Design review of the part shown in the three views and the two pictorial views. Dimensions are in mm from the part's minimum x, y and z. A direction names the side the tool comes from. Round coordinates to 2 decimals unless told otherwise and drop trailing zeros. Write each loop counter-clockwise with the first axis right and the second up, starting at its lowest first coordinate (ties: lowest second). Pieces come first, ordered by that corner, then holes. Notation, with made-up numbers: (30, 53.25) - (56, 53.25) arc R33 cw to (56, 89.25) - close; hole circle Ø5 at (25.25, 20.5). An arc over 180 degrees is marked (long way). Use one line per item in the form item = value.
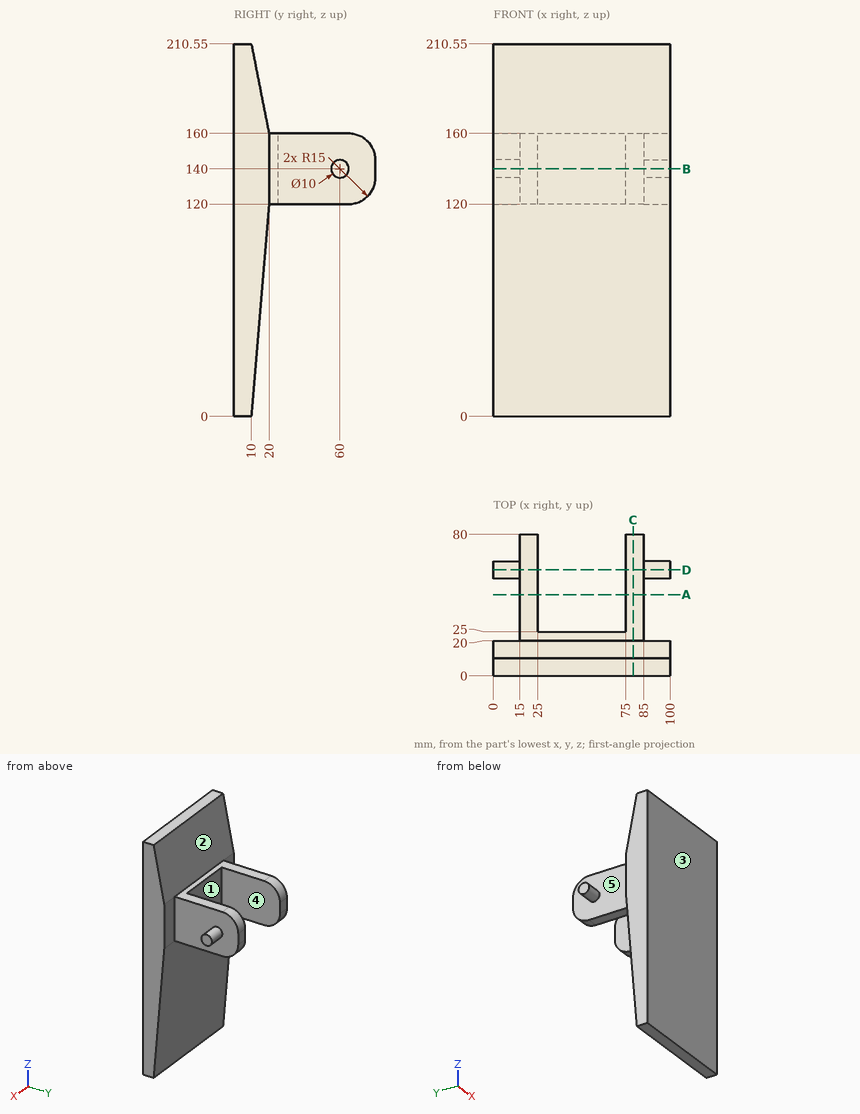
Q1. We need section C-C on x = 79. Write out the cut boundary in (y, z).
Calculated:
outline = (0, 0) - (10, 0) - (20, 120) - (65, 120) arc R15 ccw to (80, 135) - (80, 145) arc R15 ccw to (65, 160) - (20, 160) - (10, 210.55) - (0, 210.55) - close
Q2. To check wall thickness, follow line 1 along X through (y, z) = (32, 128.5); line 2 along Y through (x, z) = (50, 155.5); line 3 along Z through (x, y) = (20.5, 37). State the ranges of each line that lie inside material, in increasing order. Write a range as from..to.
Calculated:
line_1 = 15..25, 75..85
line_2 = 0..25
line_3 = 120..160
Q3. We need section A-A on y = 46. Write out the cut boundary in (x, z).
Calculated:
outline = (15, 120) - (25, 120) - (25, 160) - (15, 160) - close; (75, 120) - (85, 120) - (85, 160) - (75, 160) - close
Q4. We need section D-D on y = 60. Write out the cut boundary in (x, z).
Calculated:
outline = (0, 135) - (15, 135) - (15, 120) - (25, 120) - (25, 160) - (15, 160) - (15, 145) - (0, 145) - close; (75, 120) - (85, 120) - (85, 135) - (100, 135) - (100, 145) - (85, 145) - (85, 160) - (75, 160) - close
Q5. Machinability: for the marked faces 1 and 2, which of the approach directions +Z, -Z, +X, -X, +Y, -Y give a long, thin tool a straight path to every point of the face, cutting with its end or side? Answer none if there is none.
Calculated:
face_1 = +Z, -Z, +Y
face_2 = +Z, +X, -X, +Y
Q6. We need section B-B on z = 140. Write out the cut boundary in (x, y).
Calculated:
outline = (0, 0) - (100, 0) - (100, 20) - (85, 20) - (85, 55) - (100, 55) - (100, 65) - (85, 65) - (85, 80) - (75, 80) - (75, 25) - (25, 25) - (25, 80) - (15, 80) - (15, 65) - (0, 65) - (0, 55) - (15, 55) - (15, 20) - (0, 20) - close
Q7. Draft analysis for pull direction Y (two halves, no side actions). For the marked faces 3, 4 and 5, state which applies: released by +Y, released by -Y, zero draft, split by the parting line, or undercut.
Calculated:
face_3 = released by -Y
face_4 = zero draft
face_5 = undercut
Q8. For P1, Ø20, axis at y = 58, z = 133.5, coming from the +X side; P2, Ø22.5, axis at x = 41, y = 43.5, coming from the +Z side; P3, Ø12, axis at y = 45, z = 140, coming from the +X side; P4, Ø4.5, axis at x = 9, z = 137.5, coming from the +Y side, all flat-tipped, find the tip position at first contact; note any pin that passes through.
Calculated:
P1 = 100
P2 = through
P3 = 85
P4 = 64.99
